```python
from build123d import *

# Parameters (mm, degrees)
SKIZZE1_R                       = 18.5
AUFSATZ_LINEAR_AUSTRAGEN1_DEPTH = 65
SKIZZE2_R                       = 6
AUFSATZ_LINEAR_AUSTRAGEN2_DEPTH = 6
AUFSATZ_LINEAR_AUSTRAGEN3_DEPTH = 15


with BuildPart() as part:
    # Skizze1 → Aufsatz-Linear austragen1 (new body)
    with BuildSketch(Plane(origin=(0, 0, 0), x_dir=(0, 0, -1), z_dir=(1, 0, 0))):
        Circle(SKIZZE1_R)
    extrude(amount=AUFSATZ_LINEAR_AUSTRAGEN1_DEPTH)

    # Skizze2 → Aufsatz-Linear austragen2 (add)
    with BuildSketch(Plane.ZY):
        with Locations((0, 7)):
            Circle(SKIZZE2_R)
    extrude(amount=AUFSATZ_LINEAR_AUSTRAGEN2_DEPTH)

    # Skizze3 → Aufsatz-Linear austragen3 (add)
    with BuildSketch(Plane.ZY.offset(6)):
        with BuildLine():
            Line((-1.658312395, 9.5), (1.658312395, 9.5))
            ThreePointArc((1.658312395, 9.5), (0, 4), (-1.658312395, 9.5))
        make_face()
    extrude(amount=AUFSATZ_LINEAR_AUSTRAGEN3_DEPTH)


solid = part.part
```
Read the model definition and answer for the solid it produces. Units are mm, in the model's axes. A direction names the side the tool comes from. Give positions to 0.01 mm unless a question says otherwise; leave off trailing zeros. Loops run counter-clockwise (first coordinate to the right, second up) from the corner with the lowest first, then second, coordinate; pieces in that order, holes last.
Item 1: The part is cut by section D-D (y = 3). Write down the section's boundary in (x, z).
Item 2: Find the intervals of material crossed by line 1 along X through (y, z) = (5.5, 8); line 2 along Y through (x, z) = (-6.5, 0); line 3 along X through (y, z) = (12, 1.5), in increasing order.
Item 3: The part is cut by section C-C (y = 7). Write down the section's boundary in (x, z), and give its area (3 significant figures).
Item 4: Each of these flat-tipped pins is pushed along its axis until it touches: pin 1 Ø6 at (x, z) = (42, 10.5) entering from -Y; pin 2 Ø4 at (x, y) = (19, 7) entering from -Z; pin 3 Ø12 at (x, z) = (-3.5, -3.5) entering from +Y; pin 4 Ø8 at (y, z) = (13.5, 14) entering from +X. Where does it stop, or does it pass through?
Item 5: The part is cut by section A-A (z = 0). Write down the section's boundary in (x, y).
Item 6: The part is cut by section B-B (x = -1). Write down the section's boundary in (y, z), and give its area (3 significant figures).
Item 7: For faces 1 (the cylindrical face through (-2.96, 12.95, -0.78)), 2 (the flat face through (-13, 9.5, 0)), 3 (the flat face through (-21, 7, 0)), determine the directions among +Z, -Z, +X, -X, +Y, -Y from which every point of the face is accessible in a straight line to the end or side of a thin tool.
Taken from the geometry:
1. outline: (-6, -4.47) - (0, -4.47) - (0, -18.26) - (65, -18.26) - (65, 18.26) - (0, 18.26) - (0, 4.47) - (-6, 4.47) - close
2. line 1: x = 0 to 65
2. line 2: y = 4 to 9.5
2. line 3: x = -6 to 65
3. outline: (-21, -3) - (-6, -3) - (-6, -6) - (0, -6) - (0, -17.12) - (65, -17.12) - (65, 17.12) - (0, 17.12) - (0, 6) - (-6, 6) - (-6, 3) - (-21, 3) - close
3. area: 2,390 mm2
4. pin 1: stops at y = -16.91
4. pin 2: stops at z = -17.81
4. pin 3: stops at y = 18.5
4. pin 4: stops at x = 65
5. outline: (-21, 4) - (-6, 4) - (-6, 1) - (0, 1) - (0, -18.5) - (65, -18.5) - (65, 18.5) - (0, 18.5) - (0, 13) - (-6, 13) - (-6, 9.5) - (-21, 9.5) - close
6. outline: circle Ø12 at (7, 0)
6. area: 113 mm2
7. face 1: -X
7. face 2: +Z, -Z, -X, +Y
7. face 3: +Z, -Z, -X, +Y, -Y
